Build history of the part. All positions in model axes, mm. Face numbers are marked on the shaded views. A direction names the side the tool comes from. Round coordinates to 2 decimals unless told otherwise and drop trailing zeros. Write each loop counter-clockwise with the first axis right and the second up, starting at its lowest first coordinate (ties: lowest second). Pieces come first, ordered by that corner, then holes.
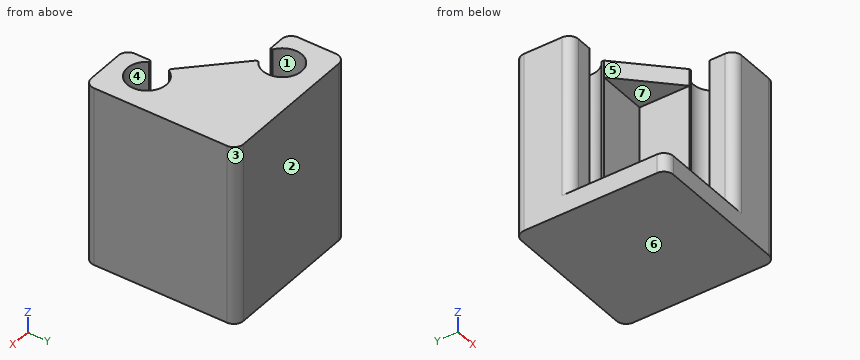
from build123d import *

# Parameters (mm, degrees)
PAD_DEPTH    = 17
SKETCH001_W  = 16
SKETCH001_H  = 16
PAD001_DEPTH = 2
PAD002_DEPTH = 1.8
FILLET_R     = 1


with BuildPart() as part:
    # Sketch → Pad (new body)
    with BuildSketch(Plane.XY):
        with BuildLine():
            Line((-10, 0), (-10, 6))
            Line((-10, 6), (6, 6))
            Line((6, 6), (6, -10))
            Line((6, -10), (0, -10))
            Line((0, -7.35), (0, -10))
            Line((0, -7.35), (0.239318, -7.35))
            ThreePointArc((0.239318, -7.35), (4.05, -6.3), (0.239318, -5.25))
            Line((0, -5.25), (0.239318, -5.25))
            Line((0, 0), (0, -5.25))
            Line((0, 0), (-5.25, 0))
            Line((-5.25, 0), (-5.25, 0.239318))
            ThreePointArc((-5.25, 0.239318), (-6.3, 4.05), (-7.35, 0.239318))
            Line((-7.35, 0), (-7.35, 0.239318))
            Line((-10, 0), (-7.35, 0))
        make_face()
    extrude(amount=PAD_DEPTH)

    # Sketch001 (on Face15 of Pad) → Pad001 (join)
    with BuildSketch(Plane(origin=(0, 0, 0), x_dir=(1, 0, 0), z_dir=(0, 0, -1))):
        with Locations((-2, 2)):
            Rectangle(SKETCH001_W, SKETCH001_H)
    extrude(amount=PAD001_DEPTH)

    # Sketch002 (on Face1 of Pad001) → Pad002 (join)
    with BuildSketch(Plane.XY.offset(17)):
        Polygon((-5.25, 0), (0, -5.25), (0, 0), align=None)
    extrude(amount=-PAD002_DEPTH)

    # Fillet
    fillet_edges = [part.edges().sort_by_distance(p)[0] for p in [
        (6, -10, 7.5),
        (6, 6, 7.5),
        (-10, 6, 7.5),
        (0, -10, 8.5),
        (-10, 0, 8.5),
        (-10, -10, -1),
    ]]
    fillet(fillet_edges, radius=FILLET_R)


solid = part.part
1) Wall check: L1, parallel to Y at x = 2, z = 7.5; L2, parallel to Z at x = -1.25, y = -0.75; L3, parallel to Z at x = -6.5, y = -7.25. Give the ranges that are in metal, low to high.
Results:
L1: y = -10 to -8.35, -4.25 to 6
L2: z = -2 to 0, 15.2 to 17
L3: z = -2 to 0
2) Pin check, flat tips, straight feed: pin 1 Ø0.5 at (x, z) = (-8.5, 11.5) entering from -Y; pin 2 Ø1.8 at (y, z) = (-8.5, 7.5) entering from -X; pin 3 Ø1.5 at (y, z) = (0, 11) entering from -X; pin 4 Ø5.5 at (x, y) = (-6.3, 2) entering from +Z. Stop position of each tip, or through.
Results:
pin 1: stops at y = 0
pin 2: stops at x = 0
pin 3: stops at x = -9.97
pin 4: stops at z = 17
3) Mould opens along X. For the marked faces 1, 2 and 3 say: released by +X, released by -X, zero draft, split by the parting line, or undercut.
Results:
face 1: undercut
face 2: zero draft
face 3: released by +X
4) Slice it at A-A (x = -4). Write the cut outline in (y, z).
Results:
outline: (-10, -2) - (6, -2) - (6, 17) - (-1.25, 17) - (-1.25, 15.2) - (0, 15.2) - (0, 0) - (-10, 0) - close
5) Which spindle directions (+Z, -Z, +X, -X, +Y, -Y) get a long thin tool onto all of the face, cutting with end or side? Do the marked faces 4, 5, 6 and 7. Say none if no direction does.
Results:
face 4: +Z
face 5: +Z, -X, -Y
face 6: -Z, +X, -X, +Y, -Y
face 7: -X, -Y
6) Slice it at C-C (z = 5.25). Write the cut outline in (x, y), plus the area to 3 significant figures.
Results:
outline: (-10, 1) arc R1 ccw to (-9, 0) - (-7.35, 0) - (-7.35, 0.24) arc R2.05 cw (long way) to (-5.25, 0.24) - (-5.25, 0) - (0, 0) - (0, -5.25) - (0.24, -5.25) arc R2.05 cw (long way) to (0.24, -7.35) - (0, -7.35) - (0, -9) arc R1 ccw to (1, -10) - (5, -10) arc R1 ccw to (6, -9) - (6, 5) arc R1 ccw to (5, 6) - (-9, 6) arc R1 ccw to (-10, 5) - close
area: 128 mm2
7) Slice it at D-D (x = -6.3). Write the cut outline in (y, z).
Results:
outline: (-10, -2) - (6, -2) - (6, 17) - (4.05, 17) - (4.05, 0) - (-10, 0) - close
8) Slice it at B-B (y = 2). Write the cut outline in (x, z), plus the area to 3 significant figures.
Results:
outline: (-10, -2) - (6, -2) - (6, 17) - (-4.25, 17) - (-4.25, 0) - (-8.35, 0) - (-8.35, 17) - (-10, 17) - close
area: 234 mm2
